Work out the finished part from the listing and answer in its coordinate system (mm). Face numbers are marked on the shaded views. A direction names the side the tool comes from. Give positions to 0.01 mm unless a question says otherwise; leave off trailing zeros. Loops run counter-clockwise (first coordinate to the right, second up) from the corner with the lowest first, then second, coordinate; pieces in that order, holes last. Notation, with made-up numbers: (67, 23) - (87, 23) arc R12 cw to (87, 46) - close; hole circle Ø3 at (24.25, 11). An arc over 180 degrees is marked (long way). Use CSV: the item, a comma, the result in double quotes.
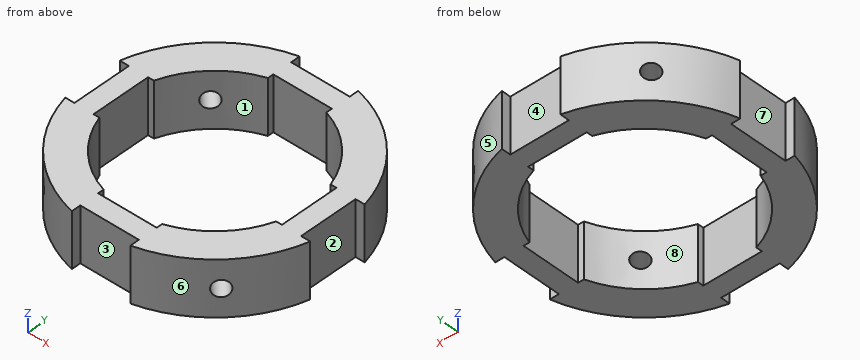
from build123d import *

# Parameters (mm, degrees)
F0_R      = 29.21
F0_R_2    = 21.59
F1_DEPTH  = 12.7
F2_W      = 13.589
F2_H      = 3.556
F2_W_2    = 3.556
F2_H_2    = 13.589
F3_DEPTH  = 25.4
F7_R      = 1.905
F8_DEPTH  = 393.7
F12_R     = 1.905
F13_DEPTH = 38.1


with BuildPart() as f1:
    # F0 (on Top) → F1 (new body)
    with BuildSketch(Plane.XY):
        Circle(F0_R)
        Circle(F0_R_2, mode=Mode.SUBTRACT)
    extrude(amount=F1_DEPTH)

    # F2 (on face) → F3 (cut)
    with BuildSketch(Plane.XY.offset(12.7)):
        with Locations((0, 20.066)):
            Rectangle(F2_W, F2_H)
        with Locations((0, 28.067)):
            Rectangle(F2_W, F2_H)
        with Locations((-20.066, 0)):
            Rectangle(F2_W_2, F2_H_2)
        with Locations((-28.067, 0)):
            Rectangle(F2_W_2, F2_H_2)
        with Locations((0, -20.066)):
            Rectangle(F2_W, F2_H)
        with Locations((0, -28.067)):
            Rectangle(F2_W, F2_H)
        with Locations((20.066, 0)):
            Rectangle(F2_W_2, F2_H_2)
        with Locations((28.067, 0)):
            Rectangle(F2_W_2, F2_H_2)
    extrude(amount=-F3_DEPTH, mode=Mode.SUBTRACT)

    # F7 (on 3pt) → F8 (cut, symmetric)
    with BuildSketch(Plane(origin=(0, 0, 0), x_dir=(0.7071067812, 0.7071067812, 0), z_dir=(0.7071067812, -0.7071067812, 0))):
        with Locations((0, 6.35)):
            Circle(F7_R)
    extrude(amount=F8_DEPTH, both=True, mode=Mode.SUBTRACT)

    # F12 (on 3pt) → F13 (cut, symmetric)
    with BuildSketch(Plane(origin=(0, 0, 0), x_dir=(-0.7071067812, 0.7071067812, 0), z_dir=(0.7071067812, 0.7071067812, 0))):
        with Locations((0, 6.35)):
            Circle(F12_R)
    extrude(amount=F13_DEPTH, both=True, mode=Mode.SUBTRACT)


solid = f1.part
Item 1: A cutting plane is placed at A-A on y = 4. Determine the outline of the cut face in (x, z), and give its area (3 significant figures).
Determined:
outline,"(-26.29, 0) - (-21.84, 0) - (-21.84, 12.7) - (-26.29, 12.7) - close; (21.84, 0) - (26.29, 0) - (26.29, 12.7) - (21.84, 12.7) - close"
area,"113 mm²"
Item 2: A cutting plane is placed at D-D on x = 18. State how many separate pieces and enclosed holes the cut face has, and give its area (3 significant figures).
Determined:
separate pieces,"2"
enclosed holes,"2"
area,"249 mm²"
Item 3: For the marked faces 1, 2, 3, 4 and 5, determine the directions among +Z, -Z, +X, -X, +Y, -Y from which every point of the face is accessible in a straight line to the end or side of a thin tool.
Determined:
face 1,"+Z, -Z"
face 2,"+Z, -Z, +X"
face 3,"+Z, -Z, -Y"
face 4,"+Z, -Z, +Y"
face 5,"+Z, -Z, +X, +Y"
Item 4: Given P1, Ø1.5, axis at y = 21, z = 9, coming from the -X side; P2, Ø2, axis at y = -10, z = 2.5, coming from the +X side; P3, Ø3, axis at x = -19.5, y = 9, coming from the +Z side; P4, Ø0.7, axis at y = -21, z = 5.5, coming from the -X side, each flat-ended and moving along its own axis, determine where each tip first touches the part or whether it passes through.
Determined:
P1,"stops at x = -21.05"
P2,"stops at x = 27.79"
P3,"stops at z = 12.7"
P4,"stops at x = -19.05"
Item 5: Find the intervals of material crossed by line 1 (X direction, y = -18.5, z = 6); line 2 (X direction, y = 5.5, z = 6.75), in increasing order.
Determined:
line 1,"x = -22.6 to -21.15, -15.85 to -11.13, 11.13 to 15.85, 21.15 to 22.6"
line 2,"x = -26.29 to -21.84, 21.84 to 26.29"
Item 6: The mould has two halves that part along X. Classify the marked faces 6, 7 and 8: pulls with the +X half, pulls with the -X half, needs draft (parallel to the pull), parting line crosses it, or undercut.
Determined:
face 6,"pulls with the +X half"
face 7,"pulls with the -X half"
face 8,"undercut"
